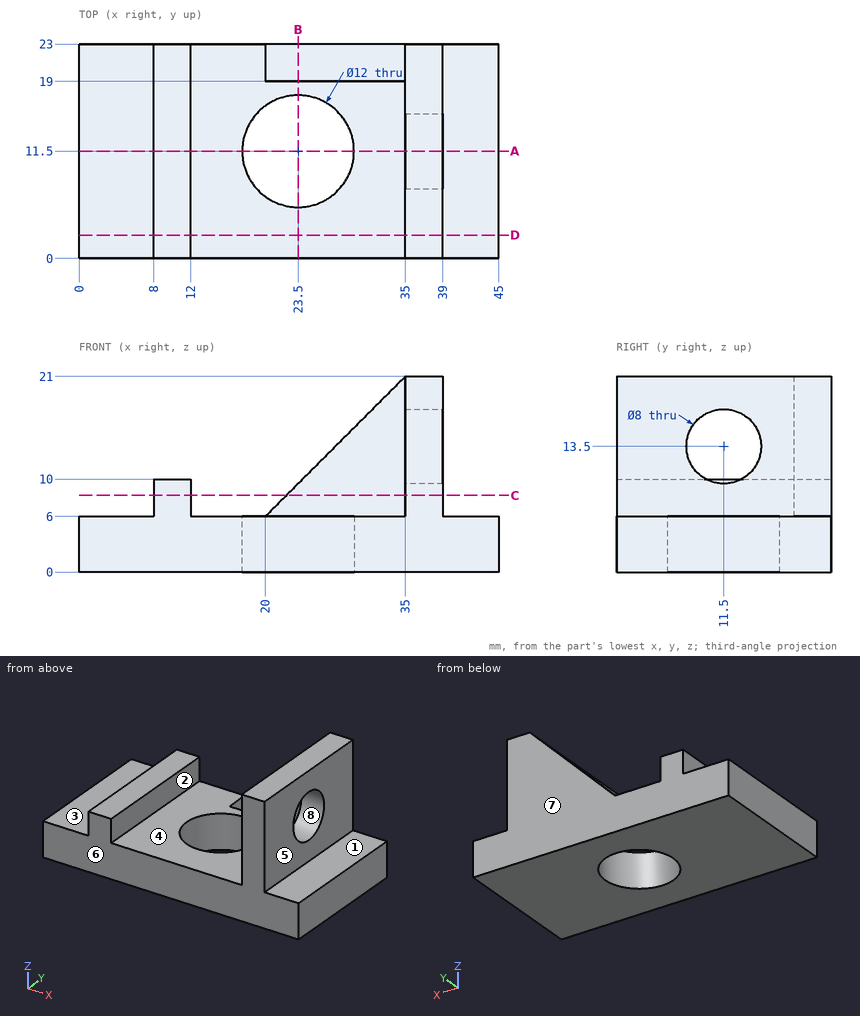
For this review, use the dimensioned drawing (mm, ordinates from the lowest corner) and the shaded views. A direction names the side the tool comes from. Give positions to 0.01 mm unless a question says otherwise; leave off trailing zeros. Write each loop counter-clockwise with the first axis right and the second up, starting at its lowest first coordinate (ties: lowest second). Pieces come first, ordered by that corner, then holes. Notation, with made-up numbers: M 62,-29.5 L 121,-29.5 A33 cw 121,0.5 Z; hole C 27,55 d10. An arc over 180 degrees is marked long. Answer as a JSON object with one key per item and string values. Group by question number.
1) We need section C-C (z = 8.25). Give the boundary of the cut face in (x, y), and give its area (3 significant figures).
2) Tool access review of the marked faces 1, 2, 3 and 4: name each direction out of +Z, -Z, +X, -X, +Y, -Y from which nothing blocks a thin tool from reaching the whole face with its end or side.
3) Mouldability with a two-part tool opening along Y and no side actions: class the marked faces 5, 6, 7 and 8 as released by +Y, released by -Y, zero draft, split by the parting line, or undercut.
4) For line 1 along Y through (x, z) = (23.5, 2.35); line 2 along X through (y, z) = (1.25, 7.5); line 3 along X through (y, z) = (21, 9), list the stretches that pass through material, from the lowest coordinate up.
5) Clearance check with flat-ended pins moving along their axes: pin 1 Ø7 at (x, y) = (23.5, 11.5) entering from -Z; pin 2 Ø1.2 at (x, y) = (9, 6) entering from +Z; pin 3 Ø1 at (x, y) = (22, 17.5) entering from +Z; pin 4 Ø1.2 at (y, z) = (9, 9) entering from -X. State where each tip first meets the part, or that it passes through.
6) We need section D-D (y = 2.5). Give the boundary of the cut face in (x, z).
7) We need section B-B (x = 23.5). Give the boundary of the cut face in (y, z), and give its area (3 significant figures).
8) We need section A-A (y = 11.5). Give the boundary of the cut face in (x, z).
Answer key:
{
 "1": {"outline": "M 8,0 L 12,0 L 12,23 L 8,23 Z; M 22.25,19 L 35,19 L 35,0 L 39,0 L 39,23 L 22.25,23 Z", "area": "235 mm²"},
 "2": {"face 1": "+Z, +X, +Y, -Y", "face 2": "+Z, +Y, -Y", "face 3": "+Z, -X, +Y, -Y", "face 4": "+Z, -Y"},
 "3": {"face 5": "zero draft", "face 6": "released by -Y", "face 7": "released by +Y", "face 8": "undercut"},
 "4": {"line 1": "y = 0 to 5.5, 17.5 to 23", "line 2": "x = 8 to 12, 35 to 39", "line 3": "x = 8 to 12, 23 to 39"},
 "5": {"pin 1": "passes through", "pin 2": "stops at z = 10", "pin 3": "stops at z = 6", "pin 4": "stops at x = 8"},
 "6": {"outline": "M 0,0 L 45,0 L 45,6 L 39,6 L 39,21 L 35,21 L 35,6 L 12,6 L 12,10 L 8,10 L 8,6 L 0,6 Z"},
 "7": {"outline": "M 0,0 L 5.5,0 L 5.5,6 L 0,6 Z; M 17.5,0 L 23,0 L 23,9.5 L 19,9.5 L 19,6 L 17.5,6 Z", "area": "80.0 mm²"},
 "8": {"outline": "M 0,0 L 17.5,0 L 17.5,6 L 12,6 L 12,10 L 8,10 L 8,6 L 0,6 Z; M 29.5,0 L 45,0 L 45,6 L 39,6 L 39,9.5 L 35,9.5 L 35,6 L 29.5,6 Z; M 35,17.5 L 39,17.5 L 39,21 L 35,21 Z"}
}
